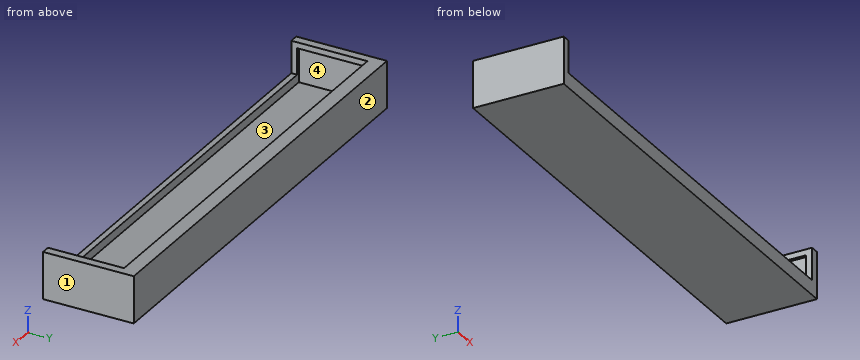
from build123d import *

# Parameters (mm, degrees)
F0_W     = 154
F0_H     = 31
F1_DEPTH = 8
F2_W     = 150
F2_H     = 27
F3_DEPTH = 6
F4_W     = 148
F4_H     = 26
F5_DEPTH = 11


with BuildPart() as f1:
    # F0 (on Top) → F1 (new body, symmetric)
    with BuildSketch(Plane.XY):
        Rectangle(F0_W, F0_H)
    extrude(amount=F1_DEPTH, both=True)

    # F2 (on Top) → F3 (cut, symmetric)
    with BuildSketch(Plane.XY):
        Rectangle(F2_W, F2_H)
    extrude(amount=F3_DEPTH, both=True, mode=Mode.SUBTRACT)

    # F4 (on face) → F5 (cut)
    with BuildSketch(Plane.XY.offset(8)):
        with Locations((0, -2.5)):
            Rectangle(F4_W, F4_H)
    extrude(amount=-F5_DEPTH, mode=Mode.SUBTRACT)


solid = f1.part
Verification items for the finished model (mm, model axes). Face numbers are marked on the shaded views. Give positions to 0.01 mm unless a question says otherwise; leave off trailing zeros. Loops run counter-clockwise (first coordinate to the right, second up) from the corner with the lowest first, then second, coordinate; pieces in that order, holes last.
1) Sectioned sample at B-B, the plane y = -6.5. Enter the section's corners in (x, z).
2) Sectioned sample at C-C, the plane x = -23.5. Enter the section's corners in (y, z).
3) Depth check by flat-ended pin: pin 1 Ø1.5 at (x, y) = (-31, -4.5) entering from +Z; pin 2 Ø2 at (x, y) = (-14.5, -14.5) entering from +Z; pin 3 Ø1 at (x, z) = (-28.5, 7) entering from -Y. Enter the tip coordinate at first touch or a pass-through.
4) Thickness scan on line 1 along X through (y, z) = (-5, 2.5); line 2 along Y through (x, z) = (29, -4.75); line 3 along Z through (x, y) = (45, -10). Record the ranges inside material, lowest first.
5) Sectioned sample at D-D, the plane z = 0.25. Enter the section's corners in (x, y).
6) Sectioned sample at A-A, the plane y = 12. Enter the section's corners in (x, z), then the cut area to 3 significant figures.
7) Draft check along Y on the marked faces 1, 2, 3 and 4. Enter one of: pulls with the +Y half, pulls with the -Y half, needs draft (parallel to the pull), parting line crosses it, or undercut.
Answers:
1. outline: (-77, -8) - (77, -8) - (77, 8) - (74, 8) - (74, 6) - (75, 6) - (75, -6) - (-75, -6) - (-75, 6) - (-74, 6) - (-74, 8) - (-77, 8) - close
2. outline: (-15.5, -8) - (15.5, -8) - (15.5, 8) - (10.5, 8) - (10.5, 6) - (13.5, 6) - (13.5, -6) - (-13.5, -6) - (-13.5, -3) - (-15.5, -3) - close
3. pin 1: stops at z = -6
3. pin 2: stops at z = -3
3. pin 3: stops at y = 10.5
4. line 1: x = -77 to -75, 75 to 77
4. line 2: y = -15.5 to -13.5, 13.5 to 15.5
4. line 3: z = -8 to -6
5. outline: (-77, -15.5) - (-74, -15.5) - (-74, -13.5) - (-75, -13.5) - (-75, 13.5) - (75, 13.5) - (75, -13.5) - (74, -13.5) - (74, -15.5) - (77, -15.5) - (77, 15.5) - (-77, 15.5) - close
6. outline: (-77, -8) - (77, -8) - (77, 8) - (-77, 8) - close; hole (-75, -6) - (75, -6) - (75, 6) - (-75, 6) - close
6. area: 664 mm2
7. face 1: needs draft
7. face 2: pulls with the +Y half
7. face 3: undercut
7. face 4: undercut
